```python
from build123d import *

# Parameters (mm, degrees)
SKETCH2_R           = 4
BOSS_EXTRUDE1_DEPTH = 20
SKETCH3_W           = 1
SKETCH3_H           = 12
CUT_EXTRUDE2_DEPTH  = 10
CHAMFER1_SIZE       = 0.3
SKETCH4_R           = 0.75
CUT_EXTRUDE3_DEPTH  = 20


with BuildPart() as part:
    # Sketch2 → Boss-Extrude1 (new body)
    with BuildSketch(Plane(origin=(0, 0, 0), x_dir=(1, 0, 0), z_dir=(0, 1, 0))):
        with Locations(Location((0, 0, 0), (0, 0, 270))):
            Circle(SKETCH2_R)
    extrude(amount=BOSS_EXTRUDE1_DEPTH)

    # Sketch3 → Cut-Extrude2 (cut, symmetric)
    with BuildSketch(Plane.XY):
        with Locations((3.5, 14)):
            Rectangle(SKETCH3_W, SKETCH3_H)
    extrude(amount=CUT_EXTRUDE2_DEPTH, both=True, mode=Mode.SUBTRACT)

    # Chamfer1
    chamfer1_edges = [part.edges().sort_by_distance(p)[0] for p in [
        (-3.645751311, 20, -1.645751311),
    ]]
    chamfer(chamfer1_edges, length=CHAMFER1_SIZE)

    # Sketch4 → Cut-Extrude3 (cut)
    with BuildSketch(Plane(origin=(0, 20, 0), x_dir=(1, 0, 0), z_dir=(0, 1, 0))):
        with Locations(Location((0, 0, 0), (0, 0, 270))):
            Circle(SKETCH4_R)
    extrude(amount=-CUT_EXTRUDE3_DEPTH, mode=Mode.SUBTRACT)


solid = part.part
```
Work out the finished part from the listing and answer in its coordinate system (mm). A direction names the side the tool comes from. Give positions to 0.01 mm unless a question says otherwise; leave off trailing zeros. Loops run counter-clockwise (first coordinate to the right, second up) from the corner with the lowest first, then second, coordinate; pieces in that order, holes last. Notation, with made-up numbers: (48, -4.5) -> (84, -4.5) arc R19 ccw to (84, 9.5) -> close; hole circle Ø2 at (8, 82). An arc over 180 degrees is marked (long way). Use CSV: the item, a comma, the result in double quotes.
1. The part is cut by section C-C (y = 15.5). Write down the section's boundary in (x, z), then the cut area to 3 significant figures.
Found:
outline,"(3, -2.65) -> (3, 2.65) arc R4 ccw (long way) to start; hole circle Ø1.5 at (0, 0)"
area,"44.9 mm^2"
2. A tool of negligible diameter and unlimited length cuts with its end or side. For faces 1 (the flat face through (3, 14, 0)), 2 (the flat face through (0, 20, 1)), from which of +Z, -Z, +X, -X, +Y, -Y can it reach the whole face along a straight path? Write none if from no direction.
Found:
face 1,"+Z, -Z, +X, +Y"
face 2,"+Z, -Z, +X, -X, +Y"
3. The part is cut by section A-A (x = 0). Write down the section's boundary in (y, z), then the cut area to 3 significant figures.
Found:
outline,"(0, -4) -> (19.7, -4) -> (20, -3.7) -> (20, -0.75) -> (0, -0.75) -> close; (0, 0.75) -> (20, 0.75) -> (20, 3.7) -> (19.7, 4) -> (0, 4) -> close"
area,"130 mm^2"
4. Flat-ended cylindrical pins translate along their axes: pin 1 Ø1.4 at (x, z) = (0, 0) entering from -Y (1 decimal); pin 2 Ø4 at (y, z) = (16, -0.5) entering from +X. Find the tip coordinate at first contact, or state that the pin passes through.
Found:
pin 1,"through"
pin 2,"x = 3"
5. The part is cut by section B-B (z = 0). Write down the section's boundary in (x, y).
Found:
outline,"(-4, 0) -> (-0.75, 0) -> (-0.75, 20) -> (-3.7, 20) -> (-4, 19.7) -> close; (0.75, 0) -> (4, 0) -> (4, 8) -> (3, 8) -> (3, 20) -> (0.75, 20) -> close"
6. The mould has two halves that part along Z. Classify faces 3 (the cylindrical face through (0.225, 10.14, 0.715)), 4 (the conical face through (-3.81, 19.89, -0.13)), 5 (the flat face through (3.4, 8, 0)): +Z half, -Z half, draft (parallel to the pull), parting line (faces both ways), or undercut.
Found:
face 3,"undercut"
face 4,"parting line"
face 5,"draft"
7. Straight lines are drawn through the part: line 1 (X direction, y = 10.75, z = 0); line 2 (Z direction, x = -0.5, y = 4.5); line 3 (Z direction, x = 0.25, y = 3.25). For each, find the intervals that lie inside material, in ascending order.
Found:
line 1,"-4 to -0.75, 0.75 to 3"
line 2,"-3.97 to -0.56, 0.56 to 3.97"
line 3,"-3.99 to -0.71, 0.71 to 3.99"
